Geometry check sheet. Reference: the model listing, model coordinates, mm. A direction names the side the tool comes from. Give positions to 0.01 mm unless a question says otherwise; leave off trailing zeros. Loops run counter-clockwise (first coordinate to the right, second up) from the corner with the lowest first, then second, coordinate; pieces in that order, holes last. Notation, with made-up numbers: (-18, 20.5) -> (-2, 20.5) arc R35 cw to (-2, 54.5) -> close; hole circle Ø4 at (-7, -21). An arc over 180 degrees is marked (long way). Write item = value, one per line. Start each with the question number.
```python
from build123d import *

# Parameters (mm, degrees)
SKETCH_1_R          = 2.5
EXTRUDE_1_DEPTH     = 1.6
SKETCH_2_R          = 1.5
EXTRUDE_2_DEPTH     = 16
CUT_EXTRUDE_1_DEPTH = 1


with BuildPart() as part:
    # 草图1 → 凸台-拉伸1 (new body)
    with BuildSketch(Plane(origin=(0, 0, 0), x_dir=(1, 0, 0), z_dir=(0, 1, 0))):
        Circle(SKETCH_1_R)
    extrude(amount=EXTRUDE_1_DEPTH)

    # 草图2 → 凸台-拉伸2 (add)
    with BuildSketch(Plane(origin=(0, 1.6, 0), x_dir=(1, 0, 0), z_dir=(0, 1, 0))):
        Circle(SKETCH_2_R)
    extrude(amount=EXTRUDE_2_DEPTH)

    # 草图3 → 切除-拉伸1 (cut)
    with BuildSketch(Plane.XZ):
        with BuildLine():
            Line((-0.5, 1), (-0.5, 1.75))
            Line((-0.5, 1.75), (0.5, 1.75))
            Line((0.5, 1.75), (0.5, 1))
            ThreePointArc((0.5, 1), (0.646446609, 0.646446609), (1, 0.5))
            Line((1, 0.5), (1.75, 0.5))
            Line((1.75, 0.5), (1.75, -0.5))
            Line((1.75, -0.5), (1, -0.5))
            ThreePointArc((1, -0.5), (0.646446609, -0.646446609), (0.5, -1))
            Line((0.5, -1), (0.5, -1.75))
            Line((0.5, -1.75), (-0.5, -1.75))
            Line((-0.5, -1.75), (-0.5, -1))
            ThreePointArc((-0.5, -1), (-0.646446609, -0.646446609), (-1, -0.5))
            Line((-1, -0.5), (-1.75, -0.5))
            Line((-1.75, -0.5), (-1.75, 0.5))
            Line((-1.75, 0.5), (-1, 0.5))
            ThreePointArc((-1, 0.5), (-0.646446609, 0.646446609), (-0.5, 1))
        make_face()
    extrude(amount=-CUT_EXTRUDE_1_DEPTH, mode=Mode.SUBTRACT)


solid = part.part
```
1) Draft check along X on faces 1 (the cylindrical face through (-1.5, 9.49, -0.07)), 2 (the flat face through (0, 1.6, 2)), 3 (the flat face through (0, 0.5, 1.75)). Enter one of: released by +X, released by -X, zero draft, split by the parting line, or undercut.
2) Section check A-A (z = 0). Enter the section's corners in (x, y).
3) Section check C-C (y = 14). Enter the section's corners in (x, z), plus the area to 3 significant figures.
4) Section check B-B (x = -0.1). Enter the section's corners in (y, z).
5) Tool access check on faces 4 (the flat face through (1.75, 0.5, 0)), 5 (the flat face through (1, 0, 1)). Record the directions out of +Z, -Z, +X, -X, +Y, -Y that give a thin tool (end or side, any length) a straight path to the whole face; none if there is none.
6) Depth check by flat-ended pin: pin 1 Ø0.8 at (x, y) = (1.5, 0.5) entering from -Z (3 decimals); pin 2 Ø2 at (y, z) = (3.5, 0) entering from +X; pin 3 Ø2 at (x, y) = (1.5, 8.5) entering from +Z. Enter the tip coordinate at first touch or a pass-through.
7) Thickness scan on line 1 (Z direction, x = -0.1, y = 16.75); line 2 (Y direction, x = 1.2, z = -1.8). Record the ranges inside material, lowest first.
8) Section check D-D (x = -2). Enter the section's corners in (y, z).
Check result:
q1.face_1 = split by the parting line
q1.face_2 = zero draft
q1.face_3 = undercut
q2.outline = (-2.5, 0) -> (-1.75, 0) -> (-1.75, 1) -> (1.75, 1) -> (1.75, 0) -> (2.5, 0) -> (2.5, 1.6) -> (1.5, 1.6) -> (1.5, 17.6) -> (-1.5, 17.6) -> (-1.5, 1.6) -> (-2.5, 1.6) -> close
q3.outline = circle Ø3 at (0, 0)
q3.area = 7.07 mm2
q4.outline = (0, -2.5) -> (1.6, -2.5) -> (1.6, -1.5) -> (17.6, -1.5) -> (17.6, 1.5) -> (1.6, 1.5) -> (1.6, 2.5) -> (0, 2.5) -> (0, 1.75) -> (1, 1.75) -> (1, -1.75) -> (0, -1.75) -> close
q5.face_4 = -Y
q5.face_5 = +Z, -Z, +X, -X, -Y
q6.pin_1 = -2.245
q6.pin_2 = 1.5
q6.pin_3 = 1.41
q7.line_1 = -1.5 to 1.5
q7.line_2 = 0 to 1.6
q8.outline = (0, -1.5) -> (1.6, -1.5) -> (1.6, 1.5) -> (0, 1.5) -> close
